For this review, take the finished solid that the model builds, in its own axes (mm). Face numbers are marked on the shaded views. A direction names the side the tool comes from. Round coordinates to 2 decimals unless told otherwise and drop trailing zeros. Write each loop counter-clockwise with the first axis right and the second up, starting at its lowest first coordinate (ties: lowest second). Pieces come first, ordered by that corner, then holes. Notation, with made-up numbers: (-25.5, 32.25) -> (7.5, 32.25) arc R26 cw to (7.5, 68.25) -> close; hole circle Ø7 at (-1.5, 22.5). An arc over 180 degrees is marked (long way). Answer as CSV lines item,"result". Start each with the question number.
Item 1: Take a section at C-C on y = -12. Give the boundary of the cut face in (x, z).
Item 2: Machinability: for the marked faces 1, 2, 3 and 4, which of the approach directions +Z, -Z, +X, -X, +Y, -Y give a long, thin tool a straight path to every point of the face, cutting with its end or side? Answer none if there is none.
Item 3: For pin 1 Ø20.5 at (x, z) = (-1.5, 63.5) entering from +Y; pin 2 Ø3 at (x, y) = (4.5, 19) entering from -Z; pin 3 Ø3 at (x, z) = (-4.5, 19.5) entering from +Y, all flat-tipped, find the tip position at first contact; note any pin that passes through.
Item 4: Wall thickness on probe 1 along Y at (x, z) = (11, 60.5); probe 2 along Z at (x, y) = (-1.5, 1): over which ranges is each line inside the solid? List them lowest first. Write a range as from..to.
Item 5: Take a section at A-A on z = 57. Give the boundary of the cut face in (x, y), then the cut area to 3 significant figures.
Item 6: Take a section at B-B on x = 3. Give the boundary of the cut face in (y, z), then the cut area to 3 significant figures.
Item 7: Take a section at D-D on x = 9.5. Give the boundary of the cut face in (y, z).
Item 8: Mouldability with a two-part tool opening along X and no side actions: class the marked faces 5, 6, 7 and 8 as +X half, -X half, draft (parallel to the pull), parting line (faces both ways), or undercut.
```python
from build123d import *

# Parameters (mm, degrees)
F1_DEPTH    = 75
F3_DEPTH    = 41.701
F4_W        = 41.7
F4_H        = 58.972705551
F5_DEPTH    = 15
F6_R        = 11.05
F7_DEPTH    = 7
F8_R        = 4.25
F9_DEPTH    = 61.034008589
F10_SIZE    = 8
F12_C1_SIZE = 5
F12_C2_SIZE = 5
F12_C3_SIZE = 5
F12_C4_SIZE = 5
F13_SIZE    = 8


with BuildPart() as f1:
    # F0 (on Top) → F1 (new body)
    with BuildSketch(Plane.XY):
        Polygon((20.85, 20.85), (0, 20.85), (-20.85, 20.85), (-20.85, 0), (-20.85, -20.85), (0, -20.85), (20.85, -20.85), (20.85, 0), align=None)
        Polygon((-12.85, 12.85), (0, 12.85), (12.85, 12.85), (12.85, 0), (12.85, -12.85), (0, -12.85), (-12.85, -12.85), (-12.85, 0), align=None, mode=Mode.SUBTRACT)
    extrude(amount=F1_DEPTH)

    # F2 (on face) → F3 (cut, through all)
    with BuildSketch(Plane(origin=(-20.85, 0, 0), x_dir=(0, -1, 0), z_dir=(-1, 0, 0))):
        Polygon((-20.85, 0), (20.85, 0), (-20.85, 41.7), align=None)
    extrude(amount=-F3_DEPTH, mode=Mode.SUBTRACT)

    # F4 (on face) → F5 (join)
    with BuildSketch(Plane(origin=(0, -10.425, 10.425), x_dir=(1, 0, 0), z_dir=(0, 0.7071067812, -0.7071067812))):
        with Locations((0, -14.7431763877)):
            Rectangle(F4_W, F4_H)
    extrude(amount=F5_DEPTH)

    # F6 (on face) → F7 (cut)
    with BuildSketch(Plane(origin=(0, 0.1816017178, -0.1816017178), x_dir=(1, 0, 0), z_dir=(0, 0.7071067812, -0.7071067812))):
        with Locations((0, -14.7431763877)):
            Circle(F6_R)
    extrude(amount=-F7_DEPTH, mode=Mode.SUBTRACT)

    # F8 (on face) → F9 (cut, through all)
    with BuildSketch(Plane(origin=(0, -4.7681457505, 4.7681457505), x_dir=(1, 0, 0), z_dir=(0, 0.7071067812, -0.7071067812))):
        with Locations((0, -14.7431763877)):
            Circle(F8_R)
    extrude(amount=-F9_DEPTH, mode=Mode.SUBTRACT)

    # F10
    f10_edges = [f1.edges().sort_by_distance(p)[0] for p in [
        (-20.85, -20.85, 37.5),
        (20.85, -20.85, 37.5),
        (20.85, 20.85, 58.35),
        (-20.85, 20.85, 58.35),
    ]]
    chamfer(f10_edges, length=F10_SIZE)

    # F12: chamfer of 5 on 4 edges, made by hand

    # F12_c1
    f12_c1_edges = [f1.edges().sort_by_distance(p)[0] for p in [
        (0, 31.4566017178, 31.0933982822),
    ]]
    chamfer(f12_c1_edges, length=F12_C1_SIZE)

    # F12_c2
    f12_c2_edges = [f1.edges().sort_by_distance(p)[0] for p in [
        (-20.85, 8.8388347648, 8.4756313292),
    ]]
    chamfer(f12_c2_edges, length=F12_C2_SIZE)

    # F12_c3
    f12_c3_edges = [f1.edges().sort_by_distance(p)[0] for p in [
        (20.85, 8.8388347648, 8.4756313292),
    ]]
    chamfer(f12_c3_edges, length=F12_C3_SIZE)

    # F12_c4
    f12_c4_edges = [f1.edges().sort_by_distance(p)[0] for p in [
        (0, -10.2433982822, -10.6066017178),
    ]]
    chamfer(f12_c4_edges, length=F12_C4_SIZE)

    # F13
    f13_edges = [f1.edges().sort_by_distance(p)[0] for p in [
        (20.85, 24.385534, 38.164466),
        (-20.85, 24.385534, 38.164466),
    ]]
    chamfer(f13_edges, length=F13_SIZE)


solid = f1.part
```
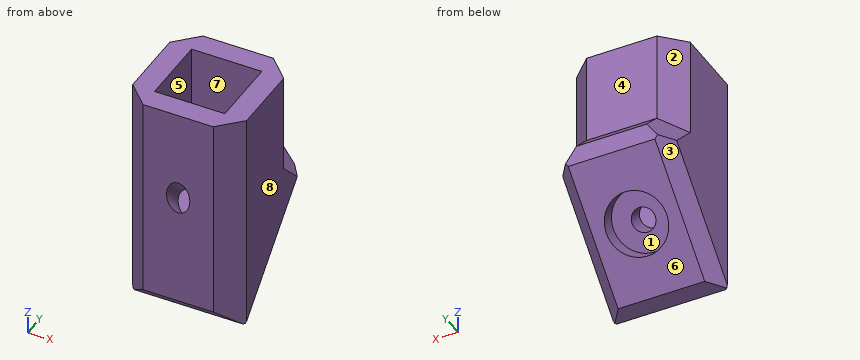
Output values:
1,outline,"(-20.85, -5.29) -> (-19.59, -7.07) -> (19.59, -7.07) -> (20.85, -5.29) -> (20.85, 75) -> (12.85, 75) -> (12.85, 8.85) -> (-12.85, 8.85) -> (-12.85, 75) -> (-20.85, 75) -> close"
2,face 1,"none"
2,face 2,"+Z, -X, +Y"
2,face 3,"-Z, -X, +Y"
2,face 4,"+Z, +X, -X, +Y"
3,pin 1,"stops at y = 20.85"
3,pin 2,"stops at z = 17.22"
3,pin 3,"stops at y = 21.36"
4,probe 1,"y = -20.85..-12.85, 12.85..20.85"
4,probe 2,"z = 0.64..4.37, 10.54..14.23"
5,outline,"(-20.85, -12.85) -> (-12.85, -20.85) -> (12.85, -20.85) -> (20.85, -12.85) -> (20.85, 12.85) -> (12.85, 20.85) -> (-12.85, 20.85) -> (-20.85, 12.85) -> close; hole (-12.85, -12.85) -> (12.85, -12.85) -> (12.85, 12.85) -> (-12.85, 12.85) -> close"
5,area,"950 mm^2"
6,outline,"(-20.85, 0) -> (-13.78, -7.07) -> (-6.71, -7.07) -> (3.09, 2.72) -> (-1.86, 7.67) -> (3.53, 13.06) -> (-2.13, 18.72) -> (-12.85, 8) -> (-12.85, 29.44) -> (-20.85, 37.44) -> close; (-20.85, 45.96) -> (-12.85, 37.96) -> (-12.85, 75) -> (-20.85, 75) -> close; (2.13, 22.98) -> (7.79, 17.32) -> (13.18, 22.71) -> (18.13, 17.76) -> (27.92, 27.56) -> (27.92, 34.63) -> (20.85, 41.7) -> (20.85, 75) -> (12.85, 75) -> (12.85, 33.7) -> close"
6,area,"1,460 mm^2"
7,outline,"(-20.85, 0) -> (-13.78, -7.07) -> (-6.71, -7.07) -> (6.62, 6.25) -> (1.67, 11.2) -> (9.65, 19.18) -> (14.6, 14.23) -> (27.92, 27.56) -> (27.92, 34.63) -> (20.85, 41.7) -> (20.85, 75) -> (12.85, 75) -> (12.85, 33.7) -> (-12.85, 8) -> (-12.85, 75) -> (-20.85, 75) -> close"
8,face 5,"undercut"
8,face 6,"draft"
8,face 7,"undercut"
8,face 8,"+X half"
